Verification items for the finished model (mm, model axes). A direction names the side the tool comes from. Give positions to 0.01 mm unless a question says otherwise; leave off trailing zeros. Loops run counter-clockwise (first coordinate to the right, second up) from the corner with the lowest first, then second, coordinate; pieces in that order, holes last. Notation, with made-up numbers: M 3.5,6 L 49.5,6 A21 cw 49.5,22 Z; hole C -3,9 d9. An arc over 180 degrees is marked long. Put each result on its own line as item: value. Start each with the question number.
from build123d import *

# Parameters (mm, degrees)
SKETCH1_W           = 98.425
SKETCH1_H           = 196.85
BOSS_EXTRUDE1_DEPTH = 41.275
CUT_EXTRUDE1_START  = -98.425
SKETCH2_W           = 12.7
SKETCH2_H           = 25.4
CUT_EXTRUDE1_DEPTH  = 95.885


with BuildPart() as part:
    # Sketch1 → Boss-Extrude1 (new body)
    with BuildSketch(Plane(origin=(0, 0, 0), x_dir=(1, 0, 0), z_dir=(0, 1, 0))):
        with Locations((49.2125, 98.425)):
            Rectangle(SKETCH1_W, SKETCH1_H)
    extrude(amount=BOSS_EXTRUDE1_DEPTH)

    # Sketch2 → Cut-Extrude1 (cut)
    with BuildSketch(Plane(origin=(98.425, 0, 0), x_dir=(0, 0, -1), z_dir=(1, 0, 0)).offset(CUT_EXTRUDE1_START)):
        with Locations((6.35, 28.575)):
            Rectangle(SKETCH2_W, SKETCH2_H)
    extrude(amount=CUT_EXTRUDE1_DEPTH, mode=Mode.SUBTRACT)


solid = part.part
Q1. Set-up check for faces 1 (the face through (98.425, 20, -97)), 2 (the face through (95.885, 29, -6)): record each of +Z, -Z, +X, -X, +Y, -Y from which the full face is reachable in a straight line by a thin tool's end or side.
Q2. Go/stop test with flat-tipped pins: pin 1 (2 mm diameter, centred on y = 10, z = -142, fed in from -X); pin 2 (4 mm diameter, centred on x = 42, z = -3.5, fed in from +Y) (3 decimals); pin 3 (6 mm diameter, centred on x = 71, y = 30, fed in from +Z); pin 4 (4 mm diameter, centred on y = 28, z = -4, fed in from -X) (3 decimals). Record where each tip stops, or that it passes through.
Q3. Scan lines: L1, parallel to Z at x = 83.5, y = 17; L2, parallel to Y at x = 25, z = -10.5 (3 decimals). Record each from-to range of solid material in increasing order.
Q4. Cross-section at B-B, the plane x = 19.5. Record the boundary of the cut face in (y, z) (3 decimals).
Q5. Cross-section at A-A, the plane y = 36. Record the boundary of the cut face in (x, z) (3 decimals), then the cut area to 3 significant figures.
Ans:
1. face 1: +Z, -Z, +X, +Y, -Y
1. face 2: +Z, -X, +Y
2. pin 1: stops at x = 0
2. pin 2: stops at y = 15.875
2. pin 3: stops at z = -12.7
2. pin 4: stops at x = 95.885
3. L1: z = -196.85 to -12.7
3. L2: y = 0 to 15.875
4. outline: M 0,-196.85 L 41.275,-196.85 L 41.275,-12.7 L 15.875,-12.7 L 15.875,0 L 0,0 Z
5. outline: M 0,-196.85 L 98.425,-196.85 L 98.425,0 L 95.885,0 L 95.885,-12.7 L 0,-12.7 Z
5. area: 18,200 mm^2
